Verification items for the finished model (mm, model axes). Face numbers are marked on the shaded views. A direction names the side the tool comes from. Round coordinates to 2 decimals unless told otherwise and drop trailing zeros. Order: outer loops, then holes, each group sorted by start corner. A loop starts at its lowest first (then second) coordinate and runs counter-clockwise, first axis right, second up. Notation, with made-up numbers: (65.5, 43.25) -> (69.5, 43.25) arc R17 cw to (69.5, 69.25) -> close; hole circle Ø4 at (36, 8). An arc over 180 degrees is marked (long way). Put each result on its own line as item: value.
from build123d import *

# Parameters (mm, degrees)
BOSS_EXTRUDE1_DEPTH   = 9.525
FILLET1_R             = 0.396875
FILLET3_RADIUS        = 5.55625
FILLET3_LENGTH        = 9.525
FILLET4_RADIUS        = 4.7625
FILLET4_LENGTH        = 4.7625
F_4_CLEARANCE_HOLE1_D = 3.2639


with BuildPart() as part:
    # Sketch1 → Boss-Extrude1 (new body)
    with BuildSketch(Plane(origin=(0, 0, 0), x_dir=(1, 0, 0), z_dir=(0, 1, 0))):
        Polygon((0, 0), (-7.9375, 0), (-7.9375, 9.525), (-4.773490222, 9.525), (-2.5527, 4.7625), (-1.5875, 4.7625), (-1.5875, 38.1), (3.175, 38.1), (3.175, 0), align=None)
    extrude(amount=BOSS_EXTRUDE1_DEPTH)

    # Fillet1
    fillet1_edges = [part.edges().sort_by_distance(p)[0] for p in [
        (-2.5527, 4.7625, -4.7625),
        (-1.5875, 4.7625, -4.7625),
    ]]
    fillet(fillet1_edges, radius=FILLET1_R)

    # Fillet3: full round fillet: the end face becomes a half cylinder, R = half its width
    fillet3_face = Plane((-2.38125, 4.7625, 0), x_dir=(0, -1, 0), z_dir=(0, 0, 1))  # on the end face: x along it, z out of the body
    fillet3_slab = fillet3_face.offset(-FILLET3_RADIUS / 2) * Box(FILLET3_LENGTH, 2 * FILLET3_RADIUS, FILLET3_RADIUS, mode=Mode.PRIVATE)  # the body's end, R deep
    fillet3_round = Plane((-2.38125, 4.7625, -5.55625), x_dir=(0, 0, 1), z_dir=(0, -1, 0)) * Cylinder(FILLET3_RADIUS, FILLET3_LENGTH, mode=Mode.PRIVATE)  # its axis R under the face
    add(fillet3_slab - fillet3_round, mode=Mode.SUBTRACT)

    # Fillet4: full round fillet: the end face becomes a half cylinder, R = half its width
    fillet4_face = Plane((0.79375, 4.7625, -38.1), x_dir=(1, 0, 0), z_dir=(0, 0, -1))  # on the end face: x along it, z out of the body
    fillet4_slab = fillet4_face.offset(-FILLET4_RADIUS / 2) * Box(FILLET4_LENGTH, 2 * FILLET4_RADIUS, FILLET4_RADIUS, mode=Mode.PRIVATE)  # the body's end, R deep
    fillet4_round = Plane((0.79375, 4.7625, -33.3375), x_dir=(0, 0, -1), z_dir=(1, 0, 0)) * Cylinder(FILLET4_RADIUS, FILLET4_LENGTH, mode=Mode.PRIVATE)  # its axis R under the face
    add(fillet4_slab - fillet4_round, mode=Mode.SUBTRACT)

    # #4 Clearance Hole1 (through all)
    with Locations(Plane(origin=(3.175, 0, 0), x_dir=(0, 0, -1), z_dir=(1, 0, 0))):
        with Locations((31.75, 4.7625)):
            Hole(F_4_CLEARANCE_HOLE1_D / 2)


solid = part.part
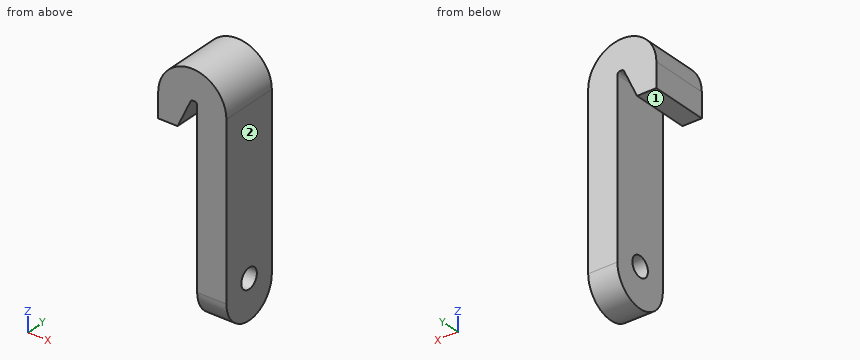
Item 1: Section check D-D on z = -20.5. Record the boundary of the cut face in (x, y) (1 decimal), then the cut area to 3 significant figures.
Check sheet entries:
outline: (-1.6, 0) -> (3.2, 0) -> (3.2, 9.5) -> (-1.6, 9.5) -> close
area: 45.4 mm^2
Item 2: Material ranges on L1, parallel to Y at x = 1.4, z = -31.75 (3 decimals); L2, parallel to X at y = 6, z = -20 (1 decimal); L3, parallel to X at y = 4.5, z = -7 (1 decimal), recorded low to high. Write a range as [from, to].
Check sheet entries:
L1: y = [0, 3.131], [6.394, 9.525]
L2: x = [-1.6, 3.2]
L3: x = [-7.9, -3.6], [-1.6, 3.2]
Item 3: Section check A-A on z = -31.75. Record the boundary of the cut face in (x, y) (1 decimal).
Check sheet entries:
outline: (-1.6, 0) -> (3.2, 0) -> (3.2, 3.1) -> (-1.6, 3.1) -> close; (-1.6, 6.4) -> (3.2, 6.4) -> (3.2, 9.5) -> (-1.6, 9.5) -> close
Item 4: Gauge pin test, flat ends, axial feed: pin 1 Ø2 at (x, y) = (-6.5, 8) entering from -Z (3 decimals); pin 2 Ø3 at (x, y) = (-3, 4) entering from -Z. Record the tip position at first contact, or that the pin passes through.
Check sheet entries:
pin 1: stops at z = -9.525
pin 2: stops at z = -38.09
Item 5: Tool access check on the marked faces 1 and 2. Record the directions out of +Z, -Z, +X, -X, +Y, -Y that give a thin tool (end or side, any length) a straight path to the whole face; none if there is none.
Check sheet entries:
face 1: -Z, -X, +Y, -Y
face 2: +Z, -Z, +X, +Y, -Y
